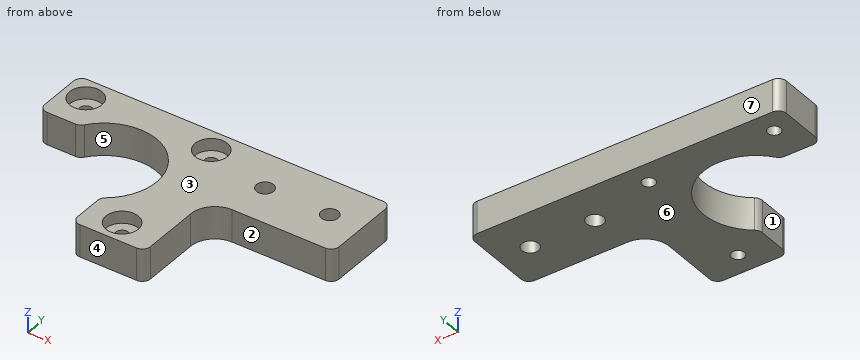
from build123d import *

# Parameters (mm, degrees)
ESQUISSE1_W             = 77
ESQUISSE1_H             = 42
BOSS_EXTRU_1_DEPTH      = 8
ESQUISSE3_R             = 4
ENL_V_MAT_EXTRU_1_DEPTH = 3
ESQUISSE4_R             = 13
ENL_V_MAT_EXTRU_2_DEPTH = 9
ESQUISSE5_W             = 28
ESQUISSE5_H             = 28
ENL_V_MAT_EXTRU_3_DEPTH = 9
ESQUISSE10_R            = 1.6
ENL_V_MAT_EXTRU_4_DEPTH = 6
ESQUISSE11_W            = 31
ESQUISSE11_H            = 22
ENL_V_MAT_EXTRU_5_DEPTH = 9
ESQUISSE12_R            = 2.1
ENL_V_MAT_EXTRU_6_DEPTH = 9
CONG_1_R                = 6
CONG_2_R                = 2


with BuildPart() as part:
    # Esquisse1 → Boss.-Extru.1 (new body)
    with BuildSketch(Plane.XY):
        with Locations((38.5, 21)):
            Rectangle(ESQUISSE1_W, ESQUISSE1_H)
    extrude(amount=BOSS_EXTRU_1_DEPTH)

    # Esquisse3 → Enlèv. mat.-Extru.1 (cut)
    with BuildSketch(Plane.XY.offset(8)):
        with Locations((5.5, 36.5)):
            Circle(ESQUISSE3_R)
        with Locations((36.5, 36.5)):
            Circle(ESQUISSE3_R)
        with Locations((36.5, 5.5)):
            Circle(ESQUISSE3_R)
    extrude(amount=-ENL_V_MAT_EXTRU_1_DEPTH, mode=Mode.SUBTRACT)

    # Esquisse4 → Enlèv. mat.-Extru.2 (cut, through all)
    with BuildSketch(Plane.XY.offset(8)):
        with Locations((21, 21)):
            Circle(ESQUISSE4_R)
    extrude(amount=-ENL_V_MAT_EXTRU_2_DEPTH, mode=Mode.SUBTRACT)

    # Esquisse5 → Enlèv. mat.-Extru.3 (cut, through all)
    with BuildSketch(Plane.XY.offset(8)):
        with Locations((14, 14)):
            Rectangle(ESQUISSE5_W, ESQUISSE5_H)
    extrude(amount=-ENL_V_MAT_EXTRU_3_DEPTH, mode=Mode.SUBTRACT)

    # Esquisse10 → Enlèv. mat.-Extru.4 (cut, through all)
    with BuildSketch(Plane.XY.offset(5)):
        with Locations((5.5, 36.5)):
            Circle(ESQUISSE10_R)
        with Locations((36.5, 36.5)):
            Circle(ESQUISSE10_R)
        with Locations((36.5, 5.5)):
            Circle(ESQUISSE10_R)
    extrude(amount=-ENL_V_MAT_EXTRU_4_DEPTH, mode=Mode.SUBTRACT)

    # Esquisse11 → Enlèv. mat.-Extru.5 (cut, through all)
    with BuildSketch(Plane.XY.offset(8)):
        with Locations((61.5, 11)):
            Rectangle(ESQUISSE11_W, ESQUISSE11_H)
    extrude(amount=-ENL_V_MAT_EXTRU_5_DEPTH, mode=Mode.SUBTRACT)

    # Esquisse12 → Enlèv. mat.-Extru.6 (cut, through all)
    with BuildSketch(Plane.XY.offset(8)):
        with Locations((53, 32)):
            Circle(ESQUISSE12_R)
        with Locations((69, 32)):
            Circle(ESQUISSE12_R)
    extrude(amount=-ENL_V_MAT_EXTRU_6_DEPTH, mode=Mode.SUBTRACT)

    # Congé1
    cong_1_edges = [part.edges().sort_by_distance(p)[0] for p in [
        (46, 22, 4),
    ]]
    fillet(cong_1_edges, radius=CONG_1_R)

    # Congé2
    cong_2_edges = [part.edges().sort_by_distance(p)[0] for p in [
        (28, 10.04554885, 4),
        (10.04554885, 28, 4),
        (0, 28, 4),
        (28, 0, 4),
        (77, 22, 4),
        (46, 0, 4),
        (0, 42, 4),
        (77, 42, 4),
    ]]
    fillet(cong_2_edges, radius=CONG_2_R)


solid = part.part
Design review of the part built by this model. Coordinates are the model's own, in mm. Face numbers are marked on the shaded views. A direction names the side the tool comes from. Give positions to 0.01 mm unless a question says otherwise; leave off trailing zeros. Order: outer loops, then holes, each group sorted by start corner. A loop starts at its lowest first (then second) coordinate and runs counter-clockwise, first axis right, second up. Notation, with made-up numbers: (73.5, 15) - (93.5, 15) arc R28 ccw to (93.5, 43) - close; hole circle Ø4 at (81, 32.5). An arc over 180 degrees is marked (long way). Use CSV: the item, a comma, the result in double quotes. Start each with the question number.
Q1. For P1, Ø1, axis at x = 47.5, y = 18, coming from the +Z side; P2, Ø3.5, axis at x = 36.5, y = 5.5, coming from the +Z side; P3, Ø6.5, axis at x = 5.5, y = 36.5, coming from the -Z side; P4, Ø3.5, axis at x = 6, z = 4.5, coming from the -Y side, all flat-tipped, find the tip position at first contact; note any pin that passes through.
Q2. Take a section at D-D (y = 36.5). State the section outline as (x, z) points.
Q3. For line 1 (Y direction, x = 5.5, z = 7.05); line 2 (Y direction, x = 69, z = 5.75); line 3 (X direction, y = 35, z = 6.5), list the stretches that pass through material, from the lowest coordinate up.
Q4. Take a section at C-C (x = 5.5). State the section outline as (y, z) points, and give its area (3 significant figures).
Q5. Take a section at B-B (z = 1.75). State the section outline as (x, y) points, and give its area (3 significant figures).
Q6. Take a section at A-A (y = 5.5). State the section outline as (x, z) points.
Q7. Machinability: for the marked faces 1, 2 and 3, which of the approach directions +Z, -Z, +X, -X, +Y, -Y give a long, thin tool a straight path to every point of the face, cutting with its end or side? Answer none if there is none.
Q8. Draft analysis for pull direction Y (two halves, no side actions). For the marked faces 4, 5, 6 and 7, state which applies: pulls with the +Y half, pulls with the -Y half, needs draft (parallel to the pull), parting line crosses it, or undercut.
Calculated:
1,P1,"passes through"
1,P2,"stops at z = 5"
1,P3,"stops at z = 0"
1,P4,"stops at y = 28"
2,outline,"(0, 0) - (3.9, 0) - (3.9, 5) - (1.5, 5) - (1.5, 8) - (0, 8) - close; (7.1, 0) - (34.9, 0) - (34.9, 5) - (32.5, 5) - (32.5, 8) - (9.5, 8) - (9.5, 5) - (7.1, 5) - close; (38.1, 0) - (77, 0) - (77, 8) - (40.5, 8) - (40.5, 5) - (38.1, 5) - close"
3,line 1,"y = 28 to 32.5, 40.5 to 42"
3,line 2,"y = 22 to 29.9, 34.1 to 42"
3,line 3,"x = 0 to 1.79, 9.21 to 32.79, 40.21 to 77"
4,outline,"(28, 0) - (34.9, 0) - (34.9, 5) - (32.5, 5) - (32.5, 8) - (28, 8) - close; (38.1, 0) - (42, 0) - (42, 8) - (40.5, 8) - (40.5, 5) - (38.1, 5) - close"
4,area,"72.0 mm²"
5,outline,"(0, 30) arc R2 ccw to (2, 28) - (9, 28) arc R2 ccw to (10.6, 28.8) arc R13 cw (long way) to (28.8, 10.6) arc R2 ccw to (28, 9) - (28, 2) arc R2 ccw to (30, 0) - (44, 0) arc R2 ccw to (46, 2) - (46, 16) arc R6 cw to (52, 22) - (75, 22) arc R2 ccw to (77, 24) - (77, 40) arc R2 ccw to (75, 42) - (2, 42) arc R2 ccw to (0, 40) - close; hole circle Ø3.2 at (5.5, 36.5); hole circle Ø3.2 at (36.5, 5.5); hole circle Ø3.2 at (36.5, 36.5); hole circle Ø4.2 at (53, 32); hole circle Ø4.2 at (69, 32)"
5,area,"1,540 mm²"
6,outline,"(28, 0) - (34.9, 0) - (34.9, 5) - (32.5, 5) - (32.5, 8) - (28, 8) - close; (38.1, 0) - (46, 0) - (46, 8) - (40.5, 8) - (40.5, 5) - (38.1, 5) - close"
7,face 1,"+Z, -Z, -X, -Y"
7,face 2,"+Z, -Z, +X, -Y"
7,face 3,"+Z, +X, -X, +Y, -Y"
8,face 4,"pulls with the -Y half"
8,face 5,"undercut"
8,face 6,"needs draft"
8,face 7,"pulls with the +Y half"
